Source: CAD feature listing. Evaluate the final solid. Frame: model axes, mm. Give positions to 0.01 mm unless a question says otherwise; leave off trailing zeros. Order: outer loops, then holes, each group sorted by start corner. A loop starts at its lowest first (then second) coordinate and runs counter-clockwise, first axis right, second up. Notation, with made-up numbers: (-35, 40.25) - (-26, 40.25) arc R26 cw to (-26, 63.25) - close; hole circle Ø3 at (39, 9.5). An arc over 180 degrees is marked (long way). One line per item, written item: value. Start each with the question number.
from build123d import *

# Parameters (mm, degrees)
SKETCH1_W           = 56
SKETCH1_H           = 56
BOSS_EXTRUDE2_DEPTH = 2
SKETCH2_R           = 7.5
SKETCH2_R_2         = 1.5
CUT_EXTRUDE1_DEPTH  = 160.818647222
SKETCH3_R           = 2.5
SKETCH3_R_2         = 1.5
CUT_EXTRUDE2_DEPTH  = 160.818647222


with BuildPart() as part:
    # Sketch1 → Boss-Extrude2 (new body)
    with BuildSketch(Plane(origin=(0, 0, 0), x_dir=(1, 0, 0), z_dir=(0, 1, 0))):
        with BuildLine():
            Line((28, 33), (28, 103))
            ThreePointArc((28, 103), (25.071067812, 110.071067812), (18, 113))
            Line((18, 113), (-18, 113))
            ThreePointArc((-18, 113), (-25.071067812, 110.071067812), (-28, 103))
            Line((-28, 103), (-28, 33))
            Line((-28, 33), (-28, 28))
            Line((-28, 28), (28, 28))
            Line((28, 28), (28, 33))
        make_face()
        Rectangle(SKETCH1_W, SKETCH1_H)
        with BuildLine():
            Line((-28, -28), (-28, 28))
            Line((-28, 28), (-33, 28))
            Line((-33, 28), (-103, 28))
            ThreePointArc((-103, 28), (-110.071067812, 25.071067812), (-113, 18))
            Line((-113, 18), (-113, -18))
            ThreePointArc((-113, -18), (-110.071067812, -25.071067812), (-103, -28))
            Line((-103, -28), (-33, -28))
            Line((-33, -28), (-28, -28))
        make_face()
        with BuildLine():
            Line((28, -33), (28, -28))
            Line((28, -28), (-28, -28))
            Line((-28, -28), (-28, -33))
            Line((-28, -33), (-28, -103))
            ThreePointArc((-28, -103), (-25.071067812, -110.071067812), (-18, -113))
            Line((-18, -113), (18, -113))
            ThreePointArc((18, -113), (25.071067812, -110.071067812), (28, -103))
            Line((28, -103), (28, -33))
        make_face()
        with BuildLine():
            Line((33, 28), (28, 28))
            Line((28, 28), (28, -28))
            Line((28, -28), (33, -28))
            Line((33, -28), (103, -28))
            ThreePointArc((103, -28), (110.071067812, -25.071067812), (113, -18))
            Line((113, -18), (113, 18))
            ThreePointArc((113, 18), (110.071067812, 25.071067812), (103, 28))
            Line((103, 28), (33, 28))
        make_face()
        with BuildLine():
            Line((33, -28), (28, -28))
            Line((28, -28), (28, -33))
            ThreePointArc((28, -33), (29.464466094, -29.464466094), (33, -28))
        make_face()
        with BuildLine():
            Line((-28, -33), (-28, -28))
            Line((-28, -28), (-33, -28))
            ThreePointArc((-33, -28), (-29.464466094, -29.464466094), (-28, -33))
        make_face()
        with BuildLine():
            Line((-33, 28), (-28, 28))
            Line((-28, 28), (-28, 33))
            ThreePointArc((-28, 33), (-29.464466094, 29.464466094), (-33, 28))
        make_face()
        with BuildLine():
            ThreePointArc((33, 28), (29.464466094, 29.464466094), (28, 33))
            Line((28, 33), (28, 28))
            Line((28, 28), (33, 28))
        make_face()
    extrude(amount=BOSS_EXTRUDE2_DEPTH)

    # Sketch2 → Cut-Extrude1 (cut, through all)
    with BuildSketch(Plane(origin=(0, 2, 0), x_dir=(1, 0, 0), z_dir=(0, 1, 0))):
        with Locations(Location((0, 0, 0), (0, 0, 270))):
            Circle(SKETCH2_R)
        with Locations(Location((-96.5, 0, 0), (0, 0, 270))):
            Circle(SKETCH2_R_2)
        with Locations(Location((-66.5, 0, 0), (0, 0, 270))):
            Circle(SKETCH2_R_2)
        with Locations(Location((-96.5, 17.5, 0), (0, 0, 270))):
            Circle(SKETCH2_R_2)
        with Locations(Location((-66.5, 17.5, 0), (0, 0, 270))):
            Circle(SKETCH2_R_2)
        with Locations(Location((-66.5, -17.5, 0), (0, 0, 90))):
            Circle(SKETCH2_R_2)
        with Locations(Location((-96.5, -17.5, 0), (0, 0, 90))):
            Circle(SKETCH2_R_2)
        with Locations(Location((0, 96.5, 0), (0, 0, 270))):
            Circle(SKETCH2_R_2)
        with Locations(Location((0, 66.5, 0), (0, 0, 270))):
            Circle(SKETCH2_R_2)
        with Locations(Location((17.5, 96.5, 0), (0, 0, 270))):
            Circle(SKETCH2_R_2)
        with Locations(Location((17.5, 66.5, 0), (0, 0, 270))):
            Circle(SKETCH2_R_2)
        with Locations(Location((-17.5, 66.5, 0), (0, 0, 90))):
            Circle(SKETCH2_R_2)
        with Locations(Location((-17.5, 96.5, 0), (0, 0, 90))):
            Circle(SKETCH2_R_2)
        with Locations(Location((96.5, 0, 0), (0, 0, 270))):
            Circle(SKETCH2_R_2)
        with Locations(Location((66.5, 0, 0), (0, 0, 270))):
            Circle(SKETCH2_R_2)
        with Locations(Location((96.5, -17.5, 0), (0, 0, 270))):
            Circle(SKETCH2_R_2)
        with Locations(Location((66.5, -17.5, 0), (0, 0, 270))):
            Circle(SKETCH2_R_2)
        with Locations(Location((66.5, 17.5, 0), (0, 0, 90))):
            Circle(SKETCH2_R_2)
        with Locations(Location((96.5, 17.5, 0), (0, 0, 90))):
            Circle(SKETCH2_R_2)
        with Locations(Location((0, -96.5, 0), (0, 0, 270))):
            Circle(SKETCH2_R_2)
        with Locations(Location((0, -66.5, 0), (0, 0, 270))):
            Circle(SKETCH2_R_2)
        with Locations(Location((-17.5, -96.5, 0), (0, 0, 270))):
            Circle(SKETCH2_R_2)
        with Locations(Location((-17.5, -66.5, 0), (0, 0, 270))):
            Circle(SKETCH2_R_2)
        with Locations(Location((17.5, -66.5, 0), (0, 0, 90))):
            Circle(SKETCH2_R_2)
        with Locations(Location((17.5, -96.5, 0), (0, 0, 90))):
            Circle(SKETCH2_R_2)
    extrude(amount=-CUT_EXTRUDE1_DEPTH, mode=Mode.SUBTRACT)

    # Sketch3 → Cut-Extrude2 (cut, through all)
    with BuildSketch(Plane(origin=(0, 2, 0), x_dir=(1, 0, 0), z_dir=(0, 1, 0))):
        with Locations(Location((-17.5, 17.5, 0), (0, 0, 270))):
            Circle(SKETCH3_R)
        with Locations(Location((17.5, 17.5, 0), (0, 0, 270))):
            Circle(SKETCH3_R)
        with Locations(Location((17.5, -17.5, 0), (0, 0, 270))):
            Circle(SKETCH3_R)
        with Locations(Location((-17.5, -17.5, 0), (0, 0, 270))):
            Circle(SKETCH3_R)
        with Locations(Location((-18.5, 0, 0), (0, 0, 270))):
            Circle(SKETCH3_R_2)
        with Locations(Location((18.5, 0, 0), (0, 0, 270))):
            Circle(SKETCH3_R_2)
        with Locations(Location((0, -18.5, 0), (0, 0, 270))):
            Circle(SKETCH3_R_2)
        with Locations(Location((0, 18.5, 0), (0, 0, 270))):
            Circle(SKETCH3_R_2)
    extrude(amount=-CUT_EXTRUDE2_DEPTH, mode=Mode.SUBTRACT)


solid = part.part
1. Contact query for flat-ended pins moving along their axis: pin 1 Ø4 at (x, z) = (17.5, 66.5) entering from +Y; pin 2 Ø1 at (y, z) = (1, 53.5) entering from -X; pin 3 Ø4.5 at (x, z) = (17.5, -17.5) entering from +Y. Output: stop coordinate, or through.
2. Section A-A on z = -81. Return the cut outline in (x, y), then the cut area to 3 significant figures.
3. Ray query, L1, parallel to Z at x = 96.5, y = 0.5; L2, parallel to X at y = 1.7, z = -75. Return the intervals inside material, ascending.
4. Section B-B on y = 0.85. Count the separate pieces of the cut face and the enclosed holes in it, then the cut area to 3 significant figures.
5. Draft query along Z for faces 1 (the cylindrical face through (30, 1, -29)), 2 (the flat face through (-27, 0, -2)), 3 (the cylindrical face through (24.99, 0.99, 110.15)), 4 (the cylindrical face through (0.33, 1.014, -7.493)). Return one class per face: pulls with the +Z half, pulls with the -Z half, needs draft (parallel to the pull), parting line crosses it, or undercut.
Data:
1. pin 1: stops at y = 2
1. pin 2: stops at x = -28
1. pin 3: passes through
2. outline: (-28, 0) - (28, 0) - (28, 2) - (-28, 2) - close
2. area: 112 mm2
3. L1: z = -28 to -19, -16 to -1.5, 1.5 to 16, 19 to 28
3. L2: x = -28 to 28
4. separate pieces: 1
4. enclosed holes: 33
4. area: 21,600 mm2
5. face 1: pulls with the -Z half
5. face 2: needs draft
5. face 3: pulls with the +Z half
5. face 4: undercut
